The model under review builds one solid part; all positions refer to its coordinate system, in mm. Face numbers are marked on the shaded views. A direction names the side the tool comes from. Round coordinates to 2 decimals unless told otherwise and drop trailing zeros. Write each loop counter-clockwise with the first axis right and the second up, starting at its lowest first coordinate (ties: lowest second). Pieces come first, ordered by that corner, then holes. Notation, with made-up numbers: (33, 1) -> (69, 1) arc R26 ccw to (69, 36) -> close; hole circle Ø3 at (-35, -36). An arc over 180 degrees is marked (long way). Answer as a JSON object with one key per item and string values. Group by question number.
1) To check wall thickness, follow probe 1 along Y at (x, z) = (0, -40) (3 decimals); probe 2 along Y at (x, z) = (50, -52); probe 3 along X at (y, z) = (-14.5, -43). State the ranges of each line that lie inside material, in increasing order. Write a range as [from, to].
2) Machinability: for the marked faces 1 and 2, which of the approach directions +Z, -Z, +X, -X, +Y, -Y give a long, thin tool a straight path to every point of the face, cutting with its end or side? Answer none if there is none.
3) We need section D-D, the plane z = -35. Write out the cut boundary in (x, y) (3 decimals).
4) Mouldability with a two-part tool opening along X and no side actions: class the marked faces 3, 4 and 5 as pulls with the +X half, pulls with the -X half, needs draft (parallel to the pull), parting line crosses it, or undercut.
5) We need section B-B, the plane z = -65. Write out the cut boundary in (x, y) (3 decimals), then the cut area to 3 significant figures.
6) We need section C-C, the plane y = 6.5. Write out the cut boundary in (x, z), then the cut area to 3 significant figures.
7) Insertion check: pin 1 Ø5 at (x, z) = (23, -64.5) entering from +Y; pin 2 Ø1.5 at (x, z) = (47, -68) entering from -Y; pin 3 Ø3 at (y, z) = (22.5, -58.5) entering from -X. Each pin has a flat end and moves straight along its axis. Give the tip position at first contact, or say it passes through.
8) We need section A-A, the plane x = 0. Write out the cut boundary in (y, z) (3 decimals).
from build123d import *
from build123d import SkipClean  # not in build123d's __all__

# Parameters (mm, degrees)
F0_R     = 15.875
F0_R_2   = 9.525
F1_DEPTH = 76.2
F2_DEPTH = 38.1
F3_DEPTH = 25.4
F4_R     = 5.08


with BuildPart() as f1:
    # F0 (on Top) → F1 (new body)
    with BuildSketch(Plane.XY):
        with BuildLine():
            ThreePointArc((10.3219202517, 26.6456110329), (23.5741330296, 16.1490209271), (28.575, 0))
            ThreePointArc((28.575, 0), (23.5741330296, -16.1490209271), (10.3219202517, -26.6456110329))
            Line((10.3219202517, -26.6456110329), (53.34, -18.8799073091))
            ThreePointArc((53.34, -18.8799073091), (31.75, 0), (53.34, 18.8799073091))
            Line((53.34, 18.8799073091), (10.3219202517, 26.6456110329))
        make_face()
        with BuildLine():
            ThreePointArc((10.3219202517, -26.6456110329), (23.5741330296, -16.1490209271), (28.575, 0))
            ThreePointArc((28.575, 0), (23.5741330296, 16.1490209271), (10.3219202517, 26.6456110329))
            ThreePointArc((10.3219202517, 26.6456110329), (-28.575, 0), (10.3219202517, -26.6456110329))
        make_face()
        Circle(F0_R, mode=Mode.SUBTRACT)
        with BuildLine():
            ThreePointArc((69.85, 0), (65.1403190341, 12.5402452129), (53.34, 18.8799073091))
            ThreePointArc((53.34, 18.8799073091), (31.75, 0), (53.34, -18.8799073091))
            ThreePointArc((53.34, -18.8799073091), (65.1403190341, -12.5402452129), (69.85, 0))
        make_face()
        with Locations((50.8, 0)):
            Circle(F0_R_2, mode=Mode.SUBTRACT)
    extrude(amount=-F1_DEPTH)

    # F0 (on Top) → F2 (cut)
    with BuildSketch(Plane.XY):
        with BuildLine():
            ThreePointArc((69.85, 0), (65.1403190341, 12.5402452129), (53.34, 18.8799073091))
            ThreePointArc((53.34, 18.8799073091), (31.75, 0), (53.34, -18.8799073091))
            ThreePointArc((53.34, -18.8799073091), (65.1403190341, -12.5402452129), (69.85, 0))
        make_face()
        with Locations((50.8, 0)):
            Circle(F0_R_2, mode=Mode.SUBTRACT)
    extrude(amount=-F2_DEPTH, mode=Mode.SUBTRACT)

    # F0 (on Top) → F3 (cut)
    with BuildSketch(Plane.XY):
        with BuildLine():
            ThreePointArc((10.3219202517, 26.6456110329), (23.5741330296, 16.1490209271), (28.575, 0))
            ThreePointArc((28.575, 0), (23.5741330296, -16.1490209271), (10.3219202517, -26.6456110329))
            Line((10.3219202517, -26.6456110329), (53.34, -18.8799073091))
            ThreePointArc((53.34, -18.8799073091), (31.75, 0), (53.34, 18.8799073091))
            Line((53.34, 18.8799073091), (10.3219202517, 26.6456110329))
        make_face()
    with SkipClean():  # cleaning this boolean's faces spoils the solid; the shape is the same uncleaned
        extrude(amount=-F3_DEPTH, mode=Mode.SUBTRACT)

    # F4
    f4_edges = [f1.edges().sort_by_distance(p)[0] for p in [
        (53.34, -18.879907, -31.75),
        (53.34, -18.879907, -57.15),
        (53.34, 18.879907, -31.75),
        (53.34, 18.879907, -57.15),
    ]]
    fillet(f4_edges, radius=F4_R)


solid = f1.part
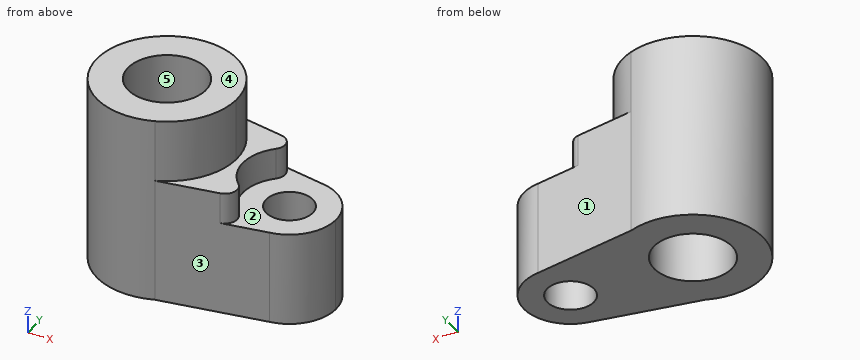
Here are the results:
{
 "1": {"probe 1": "y = [-28.575, -15.875], [15.875, 28.575]", "probe 2": "y = [-19.48, -9.49], [9.49, 19.48]", "probe 3": "x = [-24.62, -6.46], [6.46, 63.16]"},
 "2": {"face 1": "+Z, -Z, +X, +Y", "face 2": "+Z, +X"},
 "3": {"outline": "(10.322, -26.646) -> (34.806, -22.226) arc R5.08 ccw to (37.46, -13.6) arc R19.05 cw to (37.46, 13.6) arc R5.08 ccw to (34.806, 22.226) -> (10.322, 26.646) arc R28.575 ccw (long way) to start; hole circle Ø31.75 at (0, 0)"},
 "4": {"face 3": "pulls with the +X half", "face 4": "needs draft", "face 5": "undercut"},
 "5": {"outline": "(10.322, -26.646) -> (53.34, -18.88) arc R19.05 ccw to (53.34, 18.88) -> (10.322, 26.646) arc R28.575 ccw (long way) to start; hole circle Ø31.75 at (0, 0); hole circle Ø19.05 at (50.8, 0)", "area": "3,210 mm^2"},
 "6": {"outline": "(-27.83, -76.2) -> (-14.48, -76.2) -> (-14.48, 0) -> (-27.83, 0) -> close; (14.48, -76.2) -> (43.84, -76.2) -> (43.84, -38.1) -> (32.89, -38.1) -> (32.89, -25.4) -> (27.83, -25.4) -> (27.83, 0) -> (14.48, 0) -> close; (57.76, -76.2) -> (68.71, -76.2) -> (68.71, -38.1) -> (57.76, -38.1) -> close", "area": "3,120 mm^2"},
 "7": {"pin 1": "stops at y = 24.81", "pin 2": "stops at y = -20.16", "pin 3": "stops at x = -19.38"},
 "8": {"outline": "(-28.575, -76.2) -> (-15.875, -76.2) -> (-15.875, 0) -> (-28.575, 0) -> close; (15.875, -76.2) -> (28.575, -76.2) -> (28.575, 0) -> (15.875, 0) -> close"}
}
